from build123d import *

# Parameters (mm, degrees)
F12_R     = 4.7625
F13_DEPTH = 3.571875


with BuildPart() as f5:
    # F0 (on Top) → F5 section 0
    with BuildSketch(Plane.XY):
        Polygon((-31.75, 18.3308710468), (-31.75, -18.3308710468), (0, -36.6617420935), (31.75, -18.3308710468), (31.75, 18.3308710468), (0, 36.6617420935), align=None)
    # F2 (on offset) → F5 section 1
    with BuildSketch(Plane.XY.offset(50.8)):
        Polygon((-57.15, 32.9955678842), (-57.15, -32.9955678842), (0, -65.9911357684), (57.15, -32.9955678842), (57.15, 32.9955678842), (0, 65.9911357684), align=None)
    loft()

    # F5_face (on face) → F6 section 0
    with BuildSketch(Plane.XY.offset(50.8)):
        Polygon((-57.15, 32.9955678842), (-57.15, -32.9955678842), (0, -65.9911357684), (57.15, -32.9955678842), (57.15, 32.9955678842), (0, 65.9911357684), align=None)
    # F4 (on offset) → F6 section 1
    with BuildSketch(Plane.XY.offset(101.6)):
        Polygon((-31.75, 18.3308710468), (-31.75, -18.3308710468), (0, -36.6617420935), (31.75, -18.3308710468), (31.75, 18.3308710468), (0, 36.6617420935), align=None)
    loft()

    # F7 (on face) → F9 section 0
    with BuildSketch(Plane(origin=(0, 0, 0), x_dir=(1, 0, 0), z_dir=(0, 0, -1))):
        Polygon((-28.178125, 16.268648054), (-28.178125, -16.268648054), (0, -32.537296108), (28.178125, -16.268648054), (28.178125, 16.268648054), (0, 32.537296108), align=None)
    # F8 (on offset) → F9 section 1
    with BuildSketch(Plane.XY.offset(50.8)):
        Polygon((-53.578125, 30.9333448914), (-53.578125, -30.9333448914), (0, -61.8666897829), (53.578125, -30.9333448914), (53.578125, 30.9333448914), (0, 61.8666897829), align=None)
    loft(mode=Mode.SUBTRACT)

    # F8 (on offset) → F11 section 0
    with BuildSketch(Plane.XY.offset(50.8)):
        Polygon((-53.578125, 30.9333448914), (-53.578125, -30.9333448914), (0, -61.8666897829), (53.578125, -30.9333448914), (53.578125, 30.9333448914), (0, 61.8666897829), align=None)
    # F10 (on face) → F11 section 1
    with BuildSketch(Plane.XY.offset(101.6)):
        Polygon((-28.178125, 16.268648054), (-28.178125, -16.268648054), (0, -32.537296108), (28.178125, -16.268648054), (28.178125, 16.268648054), (0, 32.537296108), align=None)
    loft(mode=Mode.SUBTRACT)

    # F12 (on Top) → F13 (join)
    with BuildSketch(Plane.XY):
        Polygon((-31.7834205925, 18.3501664349), (-31.7834205925, -18.3501664349), (0, -36.7003328697), (31.7834205925, -18.3501664349), (31.7834205925, 18.3501664349), (0, 36.7003328697), align=None)
        Circle(F12_R, mode=Mode.SUBTRACT)
    extrude(amount=F13_DEPTH)


solid = f5.part
Geometry check sheet. Reference: the model listing, model coordinates, mm. Coordinates: 2 decimals unless noted, no trailing zeros. Use one line per item in the form item = value. Start each with the question number.
Item 1: Mould release check, pull along X, two halves, no side actions. Record for faces 1 (the face through (0, -7, 3.572)), 2 (the face through (-14.3, -24.5, 101.6)): +X half, -X half, draft (parallel to the pull), parting line (faces both ways), or undercut.
Item 2: Gauge pin test, flat ends, axial feed: pin 1 (10 mm diameter, centred on y = 12, z = 38.5, fed in from -X); pin 2 (10 mm diameter, centred on x = -13.5, y = 29, fed in from +Z); pin 3 (1.5 mm diameter, centred on y = 47.5, z = 13.5, fed in from -X); pin 4 (12 mm diameter, centred on y = 6, z = 82.5, fed in from -X). Record the tip position at first contact, or that the pin passes through.
Item 3: Thickness scan on probe 1 along Z at (x, y) = (-22.5, -17); probe 2 along X at (y, z) = (-31, 73); probe 3 along Z at (x, y) = (-44, 17). Record the ranges inside material, lowest first.
Computed:
q1.face_1 = undercut
q1.face_2 = draft
q2.pin_1 = -53.5
q2.pin_2 = 101.6
q2.pin_3 = through
q2.pin_4 = -44.3
q3.probe_1 = 0 to 3.57
q3.probe_2 = -38.41 to -31.26, 31.26 to 38.41
q3.probe_3 = 24.5 to 31.64, 69.96 to 77.1
